Part model, mm, in its own coordinate system. Face numbers are marked on the shaded views. A direction names the side the tool comes from. Give positions to 0.01 mm unless a question says otherwise; leave off trailing zeros. Order: outer loops, then holes, each group sorted by start corner. A loop starts at its lowest first (then second) coordinate and runs counter-clockwise, first axis right, second up. Notation, with made-up numbers: (-18, -12) - (13, -12) arc R14 ccw to (13, 3) - close; hole circle Ø10 at (35.5, 40). An arc over 180 degrees is marked (long way). Use one line per item in the form item = value. Start each with the question number.
1. Tool access for the marked faces 1, 2 and 3: list every direction of +Z, -Z, +X, -X, +Y, -Y with a clear straight run to the whole face (end or side of a thin tool).
2. Band-saw the part on B-B, the plane x = -17.5. List the corners of the cut face in (y, z), plus the area to 3 significant figures.
3. Pin check, flat tips, straight feed: P1, Ø3, axis at x = -24.5, z = 5, coming from the +Y side; P2, Ø10, axis at x = -24, z = 29, coming from the -Y side. Stop position of each tip, or through.
4. Band-saw the part on D-D, the plane x = -28. List the corners of the cut face in (y, z).
5. Band-saw the part on C-C, the plane y = -9. List the corners of the cut face in (x, z).
6. Band-saw the part on A-A, the plane z = 17.5. List the corners of the cut face in (x, y).
7. Drill centre lines: line 1 (Y direction, x = -19, z = 7); line 2 (Z direction, x = -15, y = -5.5); line 3 (Z direction, x = -21.5, y = -13). Where is each one in solid material? Low to high.
from build123d import *

# Parameters (mm, degrees)
F1_W     = 35
F1_H     = 20
F2_DEPTH = 30
F3_DEPTH = 5
F0_R     = 6.5
F6_DEPTH = 15
F7_DEPTH = 25
F8_DEPTH = 15
F9_DEPTH = 15


with BuildPart() as f2:
    # F1 (on Top) → F2 (new body)
    with BuildSketch(Plane.XY):
        with Locations((-17.5, 10)):
            Rectangle(F1_W, F1_H)
    extrude(amount=F2_DEPTH)

    # F3 (add): a face of the model
    f3_faces = [f2.faces().sort_by_distance(p)[0] for p in [
        (-17.5, 10, 30),
    ]]
    extrude(f3_faces, amount=F3_DEPTH)

    # F0 (on Front) → F6 (join)
    with BuildSketch(Plane.XZ):
        with Locations((-17.5, 17.5)):
            Circle(F0_R)
    extrude(amount=F6_DEPTH)

    # F7 (add): a face of the model
    f7_faces = [f2.faces().sort_by_distance(p)[0] for p in [
        (-34.5050252532, 0, 17.5),
    ]]
    extrude(f7_faces, amount=-F7_DEPTH)

    # F8 (add): a face of the model
    f8_faces = [f2.faces().sort_by_distance(p)[0] for p in [
        (-34.5050252532, 25, 17.5),
    ]]
    extrude(f8_faces, amount=-F8_DEPTH)

    # F9 (cut): a face of the model
    f9_faces = [f2.faces().sort_by_distance(p)[0] for p in [
        (-34.5050252532, 25, 17.5),
    ]]
    extrude(f9_faces, amount=-F9_DEPTH, mode=Mode.SUBTRACT)


solid = f2.part
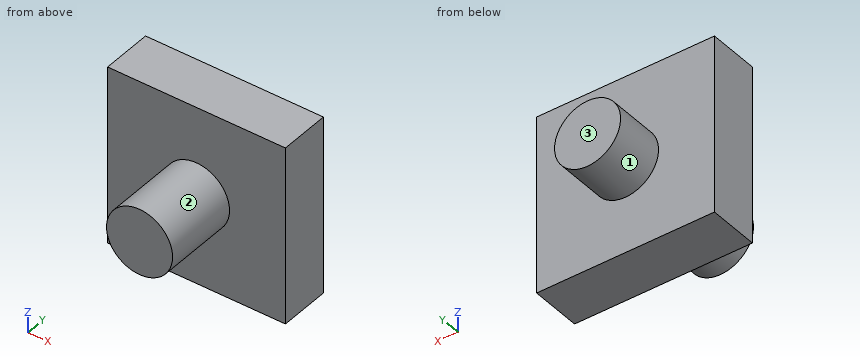
From the geometry:
q1.face_1 = +Y
q1.face_2 = -Y
q1.face_3 = +Z, -Z, +X, -X, +Y
q2.outline = (-15, 11) - (0, 11) - (0, 0) - (10, 0) - (10, 11) - (20, 11) - (20, 24) - (10, 24) - (10, 35) - (0, 35) - (0, 24) - (-15, 24) - close
q2.area = 675 mm²
q3.P1 = 10
q3.P2 = 0
q4.outline = (0, 0) - (10, 0) - (10, 35) - (0, 35) - close
q5.outline = circle Ø13 at (-17.5, 17.5)
q6.outline = (-35, 0) - (-24, 0) - (-24, -15) - (-11, -15) - (-11, 0) - (0, 0) - (0, 10) - (-11, 10) - (-11, 20) - (-24, 20) - (-24, 10) - (-35, 10) - close
q7.line_1 = 0 to 10
q7.line_2 = 11.5 to 23.5
q7.line_3 = 12.38 to 22.62
